from build123d import *

# Parameters (mm, degrees)
CUT_REVOLVE1_ANGLE = 45
CIRPATTERN1_COUNT  = 4


with BuildPart() as part:
    # Sketch1 → Revolve1 (revolve)
    with BuildSketch(Plane.XY, mode=Mode.PRIVATE) as revolve1_sk:
        Polygon((40.64, 0), (50.848864232, 38.1), (59.738864232, 38.1), (49.53, 0), align=None)
    revolve(revolve1_sk.sketch.rotate(Axis((0, 0, 0), (0, 1, 0)), 90), axis=Axis((0, 0, 0), (0, 1, 0)))

    # Sketch2 → Cut-Revolve1 (revolve, symmetric, cut)
    with BuildSketch(Plane.XY) as cut_revolve1_sk:
        Polygon((50.848864232, 38.1), (40.64, 0), (41.91, 0), (52.118864232, 38.1), align=None)
    cut_revolve1 = revolve(axis=Axis((0, 0, 0), (0, 1, 0)), revolution_arc=CUT_REVOLVE1_ANGLE / 2, mode=Mode.SUBTRACT)
    cut_revolve1 = cut_revolve1 + revolve(cut_revolve1_sk.sketch, axis=Axis((0, 0, 0), (0, -1, 0)), revolution_arc=CUT_REVOLVE1_ANGLE / 2, mode=Mode.SUBTRACT)

    # CirPattern1: Cut-Revolve1 ×4 about axis
    cirpattern1_axis = Axis((0, 38.1, 0), (0, -1, 0))
    for i in range(1, CIRPATTERN1_COUNT):
        add(cut_revolve1.rotate(cirpattern1_axis, i * 360 / CIRPATTERN1_COUNT), mode=Mode.SUBTRACT)


solid = part.part
Work out the finished part from the listing and answer in its coordinate system (mm). A direction names the side the tool comes from. Give positions to 0.01 mm unless a question says otherwise; leave off trailing zeros. Order: outer loops, then holes, each group sorted by start corner. A loop starts at its lowest first (then second) coordinate and runs counter-clockwise, first axis right, second up. Notation, with made-up numbers: M 65.25,-21 L 80.25,-21 A19 cw 80.25,-16 Z; hole C 58,-18 d4. An arc over 180 degrees is marked long. Return JSON: item names as keys, results as strings.
Q1. The mould has two halves that part along X. Classify faces 1 (the face through (31.13, 6.08, 40.6)), 2 (the face through (36.5, 0, 18.6)), 3 (the face through (42.824, 19.139, -17.738)): pulls with the +X half, pulls with the -X half, needs draft (parallel to the pull), parting line crosses it, or undercut.
Answer below:
{"face 1": "parting line crosses it", "face 2": "needs draft", "face 3": "undercut"}
Q2. Find section C-C, the plane y = 20.5. Write down the section's boundary in (x, z).
Answer below:
{"outline": "C 0,0 d110.05; hole M -43.79,-18.14 L -42.62,-17.65 A46.13 ccw -17.65,-42.62 L -18.14,-43.79 A47.4 ccw 18.14,-43.79 L 17.65,-42.62 A46.13 ccw 42.62,-17.65 L 43.79,-18.14 A47.4 ccw 43.79,18.14 L 42.62,17.65 A46.13 ccw 17.65,42.62 L 18.14,43.79 A47.4 ccw -18.14,43.79 L -17.65,42.62 A46.13 ccw -42.62,17.65 L -43.79,18.14 A47.4 ccw Z"}
Q3. Which of the six approach directions +Z, -Z, +X, -X, +Y, -Y give full straight-line access (tool end or side, diameter ignored) to faces 4 (the face through (44, 38.1, 26)), 5 (the face through (17.738, 19.139, 42.824))?
Answer below:
{"face 4": "+Z, -Z, +X, -X, +Y", "face 5": "+Y"}
Q4. Find section A-A, the plane x = 0. Write down the section's boundary in (y, z), and give its area (3 significant figures).
Answer below:
{"outline": "M 0,-49.53 L 38.1,-59.74 L 38.1,-52.12 L 0,-41.91 Z; M 0,41.91 L 38.1,52.12 L 38.1,59.74 L 0,49.53 Z", "area": "581 mm^2"}
Q5. Each of these flat-tipped pins is pushed along its axis until it touches: pin 1 (12 mm diameter, centred on x = 43.5, y = 23, fed in from +Z); pin 2 (12 mm diameter, centred on x = 24, y = 8, fed in from +Z); pin 3 (12 mm diameter, centred on y = 7.5, z = -38.5, fed in from +X). Where does it stop, or does it pass through?
Answer below:
{"pin 1": "stops at z = 41.59", "pin 2": "stops at z = 49.01", "pin 3": "stops at x = 40.42"}
Q6. Find the intervals of material crossed by line 1 along X through (y, z) = (14, 3); line 2 along Z through (x, y) = (-15.5, 12.5); line 3 along X through (y, z) = (33, -3), in increasing order. Write a range as [from, to].
Answer below:
{"line 1": "x = [-53.2, -45.56], [45.56, 53.2]", "line 2": "z = [-50.56, -42.52], [42.52, 50.56]", "line 3": "x = [-58.3, -50.66], [50.66, 58.3]"}
Q7. Find section B-B, the plane z = 0. Write down the section's boundary in (x, y).
Answer below:
{"outline": "M -59.74,38.1 L -49.53,0 L -41.91,0 L -52.12,38.1 Z; M 41.91,0 L 49.53,0 L 59.74,38.1 L 52.12,38.1 Z"}
